Autodesk Inventor part; units mm, degrees
ref_plane "Work Plane1" through (30, 0, 0) normal (0, -0.5, 0.866) x (1, 0, 0)
ref_plane "YZ Plane" through (0, 0, 0) normal (1, 0, 0) x (0, 1, 0)
ref_plane "XZ Plane" through (0, 0, 0) normal (0, 1, 0) x (-1, 0, 0)
sketch "Esquisse1" plane through (0, 0, 0) normal (0, 0, 1) x (1, 0, 0)
  line L0 (-0.6667, 0) -> (6, 0)
  line L1 (6, 0) -> (6, 1.5)
  line L2 (6, 1.5) -> (1.3067, 1.5)
  line L3 (1.3067, 1.5) -> (1, 1.5)
  line L4 (1, 1.5) -> (0, 1.5)
  line L5 (0, 1.5) -> (0, 2.75)
  line L6 (0, 2.75) -> (-3, 2.75)
  line L7 (-3, 2.75) -> (-3, 1.4434)
  line L8 (-3, 1.4434) -> (-1.5, 1.4434)
  line L9 (-1.5, 1.4434) -> (-0.6667, 0)
  line L10 (-4.8, 0) -> (7.8, 0)
  line L11 (0, -0.55) -> (0, 3.3)
  line L12 (1.3067, 1.5) -> (0, 1.5) construction
  dimension "d0" = 4.6933
  dimension "d1" = 0.3067
  dimension "d2" = 3
  dimension "d3" = 1.5
  dimension "d4" = 60
  dimension "d5" = 3
  dimension "d6" = 3
  dimension "d7" = 2.8868
  dimension "d8" = 5.5
  dimension "d19" = 6
revolve "Corps" add sketch "Esquisse1" angle 360 about axis through (-0.6667, 0, 0) along (1, 0, 0)
sketch "Esquisse2" plane through (-3, 0, 0) normal (-1, 0, 0) x (0, 0, 1)
  circle A0 centre (0, 0) radius 1.4434
  line L0 (0, -3.85) -> (0, 3.85)
  line L1 (-3.85, 0) -> (3.85, 0)
  line L2 (1.4434, 0) -> (0.7217, -1.25)
  line L3 (0.7217, -1.25) -> (-0.7217, -1.25)
  line L4 (-0.7217, -1.25) -> (-1.4434, 0)
  line L5 (-1.4434, 0) -> (-0.7217, 1.25)
  line L6 (-0.7217, 1.25) -> (0.7217, 1.25)
  line L7 (0.7217, 1.25) -> (1.4434, 0)
extrude "Rainure" add sketch "Esquisse2" against normal up to next contours L7 A0 | A0 L2 | L6 L0 A0 | A0 L0 L3 | L0 L6 A0 | A0 L3 L0 | L4 A0 | A0 L5
fillet "Congé2" radius 0.3 1 edges at (-3, -2.75, 0)
thread "Filetage"
chamfer "Chanfrein1" distance 0.3067 distance2 0.3067 1 edges at (6, -1.5, 0) measured on face at (6, -0.2617, -0.7882)
fillet "Congé1" radius 0.1 1 edges at (0, -1.5, 0)
ref_plane "Work Plane1" through (30, 0, 0) normal (0, -0.5, 0.866) x (1, 0, 0)
equation "\"d0\" = GEL"
equation "\"d1\" = GAL"
equation "\"d2\" = KOH"
equation "\"d3\" = INTI"
equation "\"d5\" = GD"
equation "\"d6\" = BDM"
equation "\"d7\" = 1.1547 * SW"
equation "\"d8\" = KOD"
equation "\"d19\" = NLG"
equation "\"d16\" = RR"
equation "\"d12\" = GEL"
equation "\"d14\" = -0.5 * SPD + 0.5 * GD"
equation "\"d15\" = GUL"
equation "\"d29\" = R"
equation "\"GD\" = NND"
equation "\"NLG\" = 6"
equation "\"GEL\" = 4.69327"
equation "\"KOD\" = 5.5"
equation "\"KOH\" = 3"
equation "\"INTI\" = 1.5"
equation "\"GAL\" = 0.61345 * PTC"
equation "\"GUL\" = 0.61345 * PTC"
equation "\"BDM\" = NND"
equation "\"SW\" = 2.5"
equation "\"RR\" = 0.3"
equation "\"SPD\" = 2.38655"
equation "\"d28\" = R"
equation "\"R\" = 0.1"
equation "\"TOA\" = 30deg"
equation "\"THREADDIA\" = 3"
equation "\"KOD1\" = KOD"
equation "\"PTC\" = 0.5"
equation "\"NND\" = 3"
equation "\"E0\" = 1.155 * SW"
equation "\"GD1\" = THREADDIA - 1.2269 * PTC"
properties part number "ANSI B18.3.1M - M3x0,5 x 6" material "Acier, doux"
Source: CAD feature listing. Evaluate the final solid. Frame: model axes, mm. A direction names the side the tool comes from. Round coordinates to 2 decimals unless told otherwise and drop trailing zeros. Loops run counter-clockwise (first coordinate to the right, second up) from the corner with the lowest first, then second, coordinate; pieces in that order, holes last. Notation, with made-up numbers: (88, -12) - (103, -12) arc R7 cw to (103, -2) - close; hole circle Ø7 at (87.25, 64). An arc over 180 degrees is marked (long way). Write item = value, one per line. Start each with the question number.
(1) Set-up query: faces 4 (the face through (-2, 1.25, 0)), 5 (the face through (0, 2, 0)), 6 (the face through (-1.369, -0.596, 2.685)). Return all of +Z, -Z, +X, -X, +Y, -Y with unobstructed straight access to the full face (end or side cutting, diameter ignored); none if empty.
(2) Section query A-A, the plane x = -2. Output: boundary loops of the cut face in (y, z).
(3) Ray query, line 1 along X through (y, z) = (2.2, -0.95); line 2 along Z through (x, y) = (-2, -1); line 3 along Y through (x, z) = (3, -0.4). Return the intervals inside material, ascending. Write a range as from..to.
(4) Section query B-B, the plane x = 1.25. Output: boundary loops of the cut face in (y, z), plus the area to 3 significant figures.
(5) Pull-direction query (Y, two-part tool) for faces 1 (the face through (-3, -1.1, 1.1)), 2 (the face through (-2.205, -0.616, 1.088)), 3 (the face through (2.86, -1.5, -0.07)); classes: +Y half, -Y half, draft (parallel to the pull), parting line (faces both ways), or undercut.
(6) Pin query (flat end, axial travel): pin 1 (3 mm diameter, centred on x = 3.5, y = 1.5, fed in from +Z); pin 2 (1 mm diameter, centred on x = 2, z = -1, fed in from +Y). Return the tip coordinate at first contact, or that it passes through.
Conclusion:
q1.face_4 = -X
q1.face_5 = +X
q1.face_6 = +X, -X
q2.outline = circle Ø5.5 at (0, 0); hole (-1.25, -0.72) - (0, -1.44) - (1.25, -0.72) - (1.25, 0.72) - (0, 1.44) - (-1.25, 0.72) - close
q3.line_1 = -3..0
q3.line_2 = -2.56..-0.87, 0.87..2.56
q3.line_3 = -1.45..1.45
q4.outline = circle Ø3 at (0, 0)
q4.area = 7.07 mm2
q5.face_1 = draft
q5.face_2 = undercut
q5.face_3 = parting line
q6.pin_1 = 1.5
q6.pin_2 = 1.41
